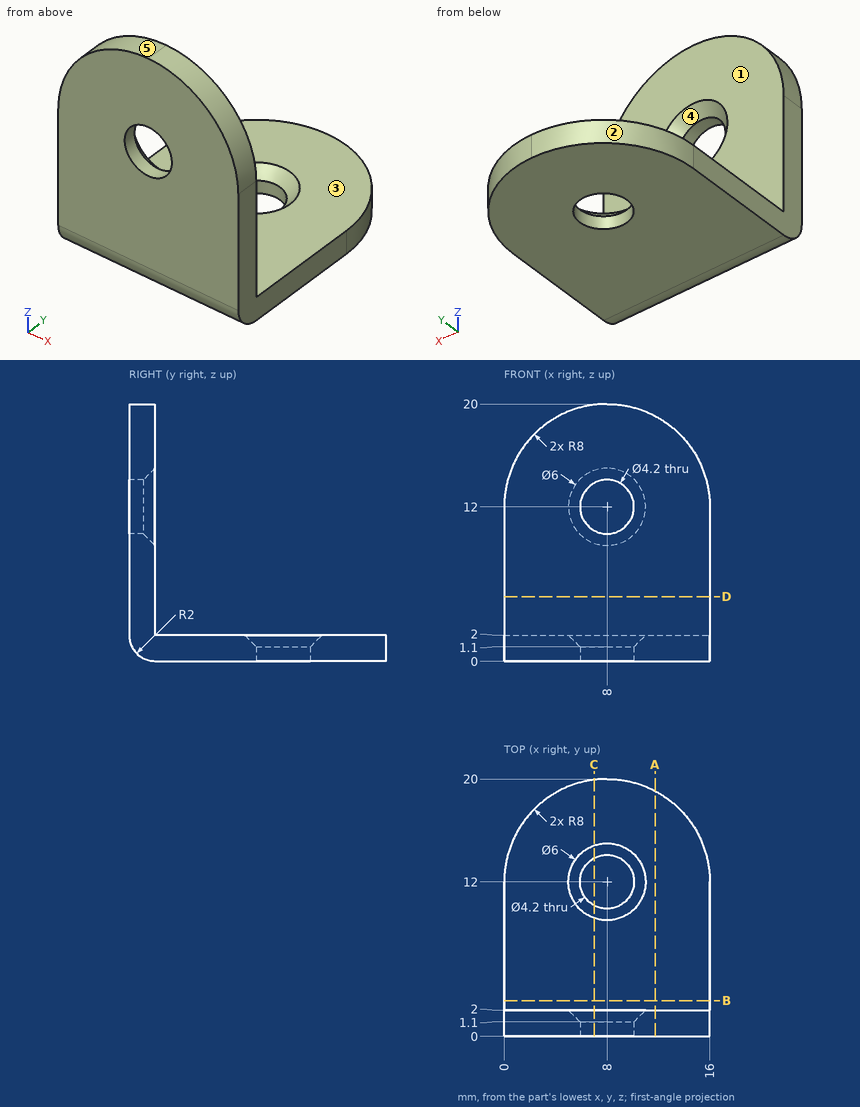
Part print with two shaded views. Sizes in mm from the minimum x, y, z corner. A direction names the side the tool comes from. Round coordinates to 2 decimals unless told otherwise and drop trailing zeros. Order: outer loops, then holes, each group sorted by start corner. A loop starts at its lowest first (then second) coordinate and runs counter-clockwise, first axis right, second up. Notation, with made-up numbers: M 18.5,-7 L 61.5,-7 A32 cw 61.5,26 Z; hole C 64.5,-25 d3. An arc over 180 degrees is marked long. Put each result on its own line as item: value. Start each with the question number.
1. Drop flat-ended pins along their axis: pin 1 (4 mm diameter, centred on x = 8, z = 12, fed in from -Y); pin 2 (5 mm diameter, centred on x = 11.5, y = 10, fed in from +Z); pin 3 (1 mm diameter, centred on x = 10.5, z = 15.5, fed in from +Y). Give the stop position or say it passes through.
2. Slice it at B-B on y = 2.75. List the corners of the cut face in (x, z), then the cut area to 3 significant figures.
3. Drill centre lines: probe 1 along X at (y, z) = (0.5, 12); probe 2 along Y at (x, z) = (12.75, 7). Where is each one in solid material? Low to high. Write a range as [from, to].
4. Two-plate mould, pull along X, no slides. Class the marked faces 3, 4 and 5: +X half, -X half, draft (parallel to the pull), parting line (faces both ways), or undercut.
5. Slice it at A-A on x = 11.75. List the corners of the cut face in (y, z).
6. Tool access for the marked faces 1 and 2: list every direction of +Z, -Z, +X, -X, +Y, -Y with a clear straight run to the whole face (end or side of a thin tool).
7. Slice it at C-C on x = 7. State how many separate pieces and enclosed holes the cut face has.
Findings:
1. pin 1: through
1. pin 2: z = 2
1. pin 3: y = 2
2. outline: M 0,0 L 16,0 L 16,2 L 0,2 Z
2. area: 32.0 mm2
3. probe 1: [0, 5.9], [10.1, 16]
3. probe 2: [0, 2]
4. face 3: draft
4. face 4: undercut
4. face 5: -X half
5. outline: M 0,2 A2 ccw 2,0 L 19.07,0 L 19.07,2 L 2,2 L 2,19.07 L 0,19.07 Z
6. face 1: +Z, +X, -X, +Y
6. face 2: +Z, -Z, -X, +Y
7. separate pieces: 3
7. enclosed holes: 0
